from build123d import *

# Parameters (mm, degrees)
SKETCH1_W           = 196
SKETCH1_H           = 336
BOSS_EXTRUDE2_DEPTH = 12
CUT_EXTRUDE1_DEPTH  = 12
CUT_EXTRUDE2_DEPTH  = 12
SKETCH7_R           = 6
CUT_EXTRUDE3_DEPTH  = 73


with BuildPart() as part:
    # Sketch1 → Boss-Extrude2 (new body)
    with BuildSketch(Plane(origin=(0, 0, 0), x_dir=(1, 0, 0), z_dir=(0, 1, 0))):
        Rectangle(SKETCH1_W, SKETCH1_H)
    extrude(amount=BOSS_EXTRUDE2_DEPTH)

    # Sketch5 → Cut-Extrude1 (cut)
    with BuildSketch(Plane(origin=(0, 12, 0), x_dir=(1, 0, 0), z_dir=(0, 1, 0))):
        with BuildLine():
            Line((10, -151.612579221), (-10, -151.612579221))
            ThreePointArc((-10, -151.612579221), (-38, -123.612579221), (-10, -95.612579221))
            Line((-10, -95.612579221), (10, -95.612579221))
            ThreePointArc((10, -95.612579221), (38, -123.612579221), (10, -151.612579221))
        make_face()
    extrude(amount=-CUT_EXTRUDE1_DEPTH, mode=Mode.SUBTRACT)

    # Sketch6 → Cut-Extrude2 (cut)
    with BuildSketch(Plane(origin=(0, 12, 0), x_dir=(1, 0, 0), z_dir=(0, 1, 0))):
        with BuildLine():
            Line((45.606081406, -5), (-44.393918594, -5))
            ThreePointArc((-44.393918594, -5), (-47.9294525, -3.535533906), (-49.393918594, 0))
            Line((-49.393918594, 0), (-49.393918594, 60))
            ThreePointArc((-49.393918594, 60), (-47.9294525, 63.535533906), (-44.393918594, 65))
            Line((-44.393918594, 65), (45.606081406, 65))
            ThreePointArc((45.606081406, 65), (49.141615312, 63.535533906), (50.606081406, 60))
            Line((50.606081406, 60), (50.606081406, 0))
            ThreePointArc((50.606081406, 0), (49.141615312, -3.535533906), (45.606081406, -5))
        make_face()
    extrude(amount=-CUT_EXTRUDE2_DEPTH, mode=Mode.SUBTRACT)

    # Sketch7 → Cut-Extrude3 (cut)
    with BuildSketch(Plane(origin=(0, 12, 0), x_dir=(1, 0, 0), z_dir=(0, 1, 0))):
        with Locations(Location((71, -118.612579221, 0), (0, 0, 270))):
            Circle(SKETCH7_R)
    extrude(amount=-CUT_EXTRUDE3_DEPTH, mode=Mode.SUBTRACT)


solid = part.part
CAD build for the part. Positions are in the model's coordinates, mm. A direction names the side the tool comes from. Coordinates: 2 decimals unless noted, no trailing zeros. Write each loop counter-clockwise with the first axis right and the second up, starting at its lowest first coordinate (ties: lowest second). Pieces come first, ordered by that corner, then holes. Notation, with made-up numbers: M 1,-11.75 L 19,-11.75 A32 ccw 19,18.25 Z; hole C 9.5,10.5 d11. An arc over 180 degrees is marked long. Return JSON: item names as keys, results as strings.
Item 1: Two-plate mould, pull along Z, no slides. Class faces 3 (the flat face through (98, 6, 2)), 4 (the cylindrical face through (72.802, 6.084, 124.336)), 5 (the flat face through (-1, 6, -168)): +Z half, -Z half, draft (parallel to the pull), parting line (faces both ways), or undercut.
Findings below:
{"face 3": "draft", "face 4": "undercut", "face 5": "-Z half"}
Item 2: Drop a flat-ended pin along its axis: pin 1 Ø3 at (x, z) = (-16.5, 46.5) entering from -Y. Give the stop position or say it passes through.
Findings below:
{"pin 1": "stops at y = 0"}
Item 3: Slice it at D-D, the plane x = -29. Write the cut outline in (y, z).
Findings below:
{"outline": "M 0,-168 L 12,-168 L 12,-65 L 0,-65 Z; M 0,5 L 12,5 L 12,103.05 L 0,103.05 Z; M 0,144.18 L 12,144.18 L 12,168 L 0,168 Z"}
Item 4: Which spindle directions (+Z, -Z, +X, -X, +Y, -Y) get a long thin tool onto all of the face, cutting with end or side? Do faces 1 (the flat face through (-1, 6, 168)), 2 (the flat face through (50.606, 6, -30)). Say none if no direction does.
Findings below:
{"face 1": "+Z, +X, -X, +Y, -Y", "face 2": "+Y, -Y"}
Item 5: Slice it at B-B, the plane z = -50.5. Write the cut outline in (x, y), and give its area (3 significant figures).
Findings below:
{"outline": "M -98,0 L -49.39,0 L -49.39,12 L -98,12 Z; M 50.61,0 L 98,0 L 98,12 L 50.61,12 Z", "area": "1,150 mm2"}
Item 6: Probe line 1 (Z direction, x = -4, y = 8.5); line 2 (X direction, y = 3.25, z = -5); line 3 (Z direction, x = 22, y = 6.5). List the from-to ranges inside material, lowest first. Write a range as from..to.
Findings below:
{"line 1": "z = -168..-65, 5..95.61, 151.61..168", "line 2": "x = -98..-49.39, 50.61..98", "line 3": "z = -168..-65, 5..98.31, 148.91..168"}
Item 7: Slice it at C-C, the plane y = 2.5. Write the cut outline in (x, z).
Findings below:
{"outline": "M -98,-168 L 98,-168 L 98,168 L -98,168 Z; hole M -49.39,-60 A5 ccw -44.39,-65 L 45.61,-65 A5 ccw 50.61,-60 L 50.61,0 A5 ccw 45.61,5 L -44.39,5 A5 ccw -49.39,0 Z; hole M -10,95.61 L 10,95.61 A28 ccw 10,151.61 L -10,151.61 A28 ccw Z; hole C 71,118.61 d12"}
Item 8: Slice it at A-A, the plane x = 71. Write the cut outline in (y, z), and give its area (3 significant figures).
Findings below:
{"outline": "M 0,-168 L 12,-168 L 12,112.61 L 0,112.61 Z; M 0,124.61 L 12,124.61 L 12,168 L 0,168 Z", "area": "3,890 mm2"}
